```python
from build123d import *

# Parameters (mm, degrees)
BOSS_EXTRUDE1_DEPTH     = 23
SKETCH2_R               = 1.5
BOSS_EXTRUDE2_DEPTH     = 5
SKETCH3_R               = 1.5
BOSS_EXTRUDE3_DEPTH     = 5
BOSS_EXTRUDE4_DEPTH     = 37
BOSS_EXTRUDE5_START     = 50
BOSS_EXTRUDE5_DEPTH     = 50
CUT_EXTRUDE1_DEPTH      = 78.86002886
CUT_EXTRUDE1_DEPTH_BACK = 78.86002886
SKETCH5_R               = 25
CUT_EXTRUDE4_DEPTH      = 20
SKETCH7_R               = 1.2
CUT_EXTRUDE6_DEPTH      = 78.86002886


with BuildPart() as part:
    # Sketch1 → Boss-Extrude1 (new body)
    with BuildSketch(Plane(origin=(0, 0, 0), x_dir=(1, 0, 0), z_dir=(0, 1, 0))):
        with BuildLine():
            ThreePointArc((0, 9.04157066), (-54.5, 0), (0, -9.04157066))
            ThreePointArc((0, -9.04157066), (54.5, 0), (0, 9.04157066))
        make_face()
    extrude(amount=BOSS_EXTRUDE1_DEPTH)

    # Sketch2 → Boss-Extrude2 (add)
    with BuildSketch(Plane(origin=(0, 0, 0), x_dir=(1, 0, 0), z_dir=(0, 1, 0))):
        with BuildLine():
            Line((-33.5, 33), (-33.5, 27.110883423))
            ThreePointArc((-33.5, 27.110883423), (-28.532848636, 27.926108329), (-23.5, 27.838821814))
            Line((-23.5, 27.838821814), (-23.5, 33))
            ThreePointArc((-23.5, 33), (-28.5, 38), (-33.5, 33))
        make_face()
        with Locations(Location((-28.5, 33, 0), (0, 0, 270))):
            Circle(SKETCH2_R, mode=Mode.SUBTRACT)
    extrude(amount=BOSS_EXTRUDE2_DEPTH)

    # Sketch3 → Boss-Extrude3 (add)
    # profile 1 of 2: a face of its own
    with BuildSketch(Plane(origin=(0, 0, 0), x_dir=(1, 0, 0), z_dir=(0, 1, 0))):
        with BuildLine():
            ThreePointArc((53.677291645, 21.033183755), (53.541166714, 28.102941176), (46.471409292, 27.966816245))
            Line((46.471409292, 27.966816245), (41.999184876, 23.318989433))
            ThreePointArc((41.999184876, 23.318989433), (45.914170974, 20.176470588), (49.205067229, 16.385356942))
            Line((49.205067229, 16.385356942), (53.677291645, 21.033183755))
        make_face()
        with Locations(Location((50.074350468, 24.5, 0), (0, 0, 270))):
            Circle(SKETCH3_R, mode=Mode.SUBTRACT)
    # profile 2 of 2: a face of its own
    with BuildSketch(Plane(origin=(0, 0, 0), x_dir=(1, 0, 0), z_dir=(0, 1, 0))):
        with BuildLine():
            Line((41.999184876, -23.318989433), (46.471409292, -27.966816245))
            ThreePointArc((46.471409292, -27.966816245), (53.541166714, -28.102941176), (53.677291645, -21.033183755))
            Line((53.677291645, -21.033183755), (49.205067229, -16.385356942))
            ThreePointArc((49.205067229, -16.385356942), (45.914170974, -20.176470588), (41.999184876, -23.318989433))
        make_face()
        with Locations(Location((50.074350468, -24.5, 0), (0, 0, 270))):
            Circle(SKETCH3_R, mode=Mode.SUBTRACT)
    extrude(amount=BOSS_EXTRUDE3_DEPTH)

    # Sketch6 → Boss-Extrude4 (add)
    with BuildSketch(Plane.XY):
        with BuildLine():
            Line((-16.5, 0), (16.5, 0))
            ThreePointArc((16.5, 0), (0, 16.5), (-16.5, 0))
        make_face()
    extrude(amount=-BOSS_EXTRUDE4_DEPTH)

    # Sketch6_2 → Boss-Extrude5 (add)
    with BuildSketch(Plane.XY.offset(BOSS_EXTRUDE5_START)):
        with BuildLine():
            Line((-16.5, 0), (16.5, 0))
            ThreePointArc((16.5, 0), (0, 16.5), (-16.5, 0))
        make_face()
    extrude(amount=-BOSS_EXTRUDE5_DEPTH)

    # Sketch4 → Cut-Extrude1 (cut, two sides: drawn at the far end of the back side and taken through both)
    with BuildSketch(Plane.XY.offset(-CUT_EXTRUDE1_DEPTH_BACK)):
        with BuildLine():
            Line((-13.5, 0), (13.5, 0))
            ThreePointArc((13.5, 0), (0, 13.5), (-13.5, 0))
        make_face()
    extrude(amount=CUT_EXTRUDE1_DEPTH + CUT_EXTRUDE1_DEPTH_BACK, mode=Mode.SUBTRACT)

    # Sketch5 → Cut-Extrude4 (cut)
    with BuildSketch(Plane(origin=(0, 0, 0), x_dir=(1, 0, 0), z_dir=(0, 1, 0))):
        with Locations(Location((-26.5, 0, 0), (0, 0, 58.667748502))):
            Circle(SKETCH5_R)
        with Locations(Location((26.5, 0, 0), (0, 0, 121.332251498))):
            Circle(SKETCH5_R)
    extrude(amount=CUT_EXTRUDE4_DEPTH, mode=Mode.SUBTRACT)

    # Sketch7 → Cut-Extrude6 (cut, through all)
    with BuildSketch(Plane(origin=(0, 0, 0), x_dir=(1, 0, 0), z_dir=(0, 1, 0))):
        with Locations(Location((-6, 0, 0), (0, 0, 270))):
            Circle(SKETCH7_R)
        with Locations(Location((6, 0, 0), (0, 0, 270))):
            Circle(SKETCH7_R)
    extrude(amount=CUT_EXTRUDE6_DEPTH, mode=Mode.SUBTRACT)


solid = part.part
```
The listing builds one solid part. Answer for the finished solid, in the listing's coordinates (mm). A direction names the side the tool comes from. Round coordinates to 2 decimals unless told otherwise and drop trailing zeros. Loops run counter-clockwise (first coordinate to the right, second up) from the corner with the lowest first, then second, coordinate; pieces in that order, holes last. Notation, with made-up numbers: (51, -34.5) - (77, -34.5) arc R26 ccw to (77, -19.5) - close; hole circle Ø1 at (-2, 88.5). An arc over 180 degrees is marked (long way). Return JSON: item names as keys, results as strings. Group by question number.
1. Consider probe 1 along X at (y, z) = (20.75, 0); probe 2 along X at (y, z) = (16, 10); probe 3 along Z at (x, y) = (-26.5, 11.75). Determine where each line is inside the solid, lowest interval first.
2. The part is cut by section D-D on x = -6. Determine the outline of the cut face in (y, z), then the cut area to 3 significant figures.
3. The part is cut by section B-B on x = 26.5. Determine the outline of the cut face in (y, z), then the cut area to 3 significant figures.
4. The part is cut by section A-A on x = -28.5. Determine the outline of the cut face in (y, z), then the cut area to 3 significant figures.
5. Which of the six approach directions +Z, -Z, +X, -X, +Y, -Y give full straight-line access (tool end or side, diameter ignored) to faces 5 (the flat face through (48, 5, -23)), 6 (the flat face through (51.47, 2.46, 18.74)), 7 (the cylindrical face through (0.363, 16.496, -29.038)), 8 (the flat face through (-33.5, 2, -30)), 9 (the flat face through (48, 5, 24))?
6. Each of these flat-tipped pins is pushed along its axis until it touches: P1, Ø2, axis at x = -6, z = 0, coming from the -Y side; P2, Ø8, axis at y = 17.5, z = 9.5, coming from the -X side; P3, Ø4, axis at x = 50, z = 23.5, coming from the +Y side; P4, Ø12, axis at y = 5.5, z = -10.5, coming from the -X side. Where does it stop, or does it pass through?
7. The part is cut by section C-C on z = -19. Determine the outline of the cut face in (x, y), then the cut area to 3 significant figures.
8. The mould has two halves that part along Z. Classify faces 1 (the flat face through (-1, 14, -37)), 2 (the flat face through (51, 0, 7)), 3 (the flat face through (44.204, 2.465, 25.61)), 4 (the flat face through (-27, 20, 0)): pulls with the +Z half, pulls with the -Z half, needs draft (parallel to the pull), parting line crosses it, or undercut.
Resolved:
{
 "1": {"probe 1": "x = -54.5 to -7.2, -4.8 to 4.8, 7.2 to 54.5", "probe 2": "x = -52.65 to -49.41, -3.59 to 3.59, 49.41 to 52.65", "probe 3": "z = -28 to -25, 25 to 28"},
 "2": {"outline": "(12.09, -37) - (15.37, -37) - (15.37, -19.07) - (23, -19.07) - (23, -1.2) - (20, -1.2) - (20, -14.31) - (12.09, -14.31) - close; (12.09, 14.31) - (20, 14.31) - (20, 1.2) - (23, 1.2) - (23, 19.07) - (15.37, 19.07) - (15.37, 50) - (12.09, 50) - close", "area": "343 mm²"},
 "3": {"outline": "(0, -28) - (23, -28) - (23, 28) - (0, 28) - (0, 25) - (20, 25) - (20, -25) - (0, -25) - close", "area": "288 mm²"},
 "4": {"outline": "(0, -38) - (5, -38) - (5, -34.5) - (0, -34.5) - close; (0, -31.5) - (5, -31.5) - (5, -27.93) - (23, -27.93) - (23, 27.93) - (0, 27.93) - (0, 24.92) - (20, 24.92) - (20, -24.92) - (0, -24.92) - close", "area": "323 mm²"},
 "5": {"face 5": "-Z, +X, +Y", "face 6": "+X, +Y, -Y", "face 7": "-Z, +Y", "face 8": "-Z, -X, +Y, -Y", "face 9": "+Z, +X, +Y"},
 "6": {"P1": "passes through", "P2": "stops at x = -53.95", "P3": "stops at y = 5", "P4": "stops at x = -54.14"},
 "7": {"outline": "(-47.07, 0) - (-42.75, 0) - (-42.75, 20) - (-10.25, 20) - (-10.25, 8.78) arc R13.5 cw to (10.25, 8.78) - (10.25, 20) - (42.75, 20) - (42.75, 0) - (51.72, 0) - (51.72, 5) - (47.07, 5) - (47.07, 23) - (5.93, 23) - (5.93, 15.4) arc R16.5 ccw to (-5.93, 15.4) - (-5.93, 23) - (-47.07, 23) - close", "area": "560 mm²"},
 "8": {"face 1": "pulls with the -Z half", "face 2": "needs draft", "face 3": "pulls with the +Z half", "face 4": "undercut"}
}
